Autodesk Inventor part; units mm, degrees
ref_plane "YZ Plane" through (0, 0, 0) normal (1, 0, 0) x (0, 1, 0)
ref_plane "XZ Plane" through (0, 0, 0) normal (0, 1, 0) x (-1, 0, 0)
ref_plane "XY Plane" through (0, 0, 0) normal (0, 0, 1) x (1, 0, 0)
sketch "Sketch1" plane through (0, 0, 0) normal (0, 0, 1) x (1, 0, 0)
  line L0 (0, 0) -> (25.4, 0)
  line L1 (25.4, 0) -> (25.4, 50.8)
  line L2 (25.4, 50.8) -> (0, 50.8)
  line L3 (0, 50.8) -> (0, 0)
  line L4 (1.5875, 1.5875) -> (23.8125, 1.5875)
  line L5 (23.8125, 1.5875) -> (23.8125, 49.2125)
  line L6 (23.8125, 49.2125) -> (1.5875, 49.2125)
  line L7 (1.5875, 49.2125) -> (1.5875, 1.5875)
  dimension "d0" = 25.4
  dimension "d1" = 50.8
  dimension "d2" = 1.5875
extrude "Extrusion1" add sketch "Sketch1" along normal blind 77.4446
sketch "Sketch2" plane through (25.4, 0, 0) normal (1, 0, 0) x (0, 0, -1)
  line L0 (0, 50.8) -> (-77.4446, 50.8)
  line L1 (-77.4446, 50.8) -> (-68.2676, 0)
  line L2 (-68.2676, 0) -> (-77.4446, 0)
  line L3 (0, 1.5875) -> (-77.4446, 1.5875)
  line L4 (-77.4446, 50.8) -> (-77.4446, 0)
  line L5 (-77.4446, 0) -> (-77.4446, 50.8)
  point P0 (0, 0)
  dimension "d5" = 10.24
sketch "Sketch3" plane through (25.4, 0, 0) normal (1, 0, 0) x (0, 0, -1)
  line L0 (0, 0) -> (0, 50.8)
  line L1 (0, 50.8) -> (-77.4446, 50.8)
  line L2 (-77.4446, 0) -> (-77.4446, 50.8)
  point P0 (-26.797, 25.4)
  dimension "d10" = 25.4
  dimension "d21" = 50.6476
hole "Hole1" at (25.4, 25.4, 26.797) direction (-1, 0, 0) diameter 28.575 depth 25.4 tip angle 118
extrude "Extrusion3" cut sketch "Sketch2" against normal blind 25.4
properties part number "ARM_029_BottomIntakeSide" material "Aluminum 6061"
Read the model definition and answer for the solid it produces. Units are mm, in the model's axes. A direction names the side the tool comes from. Coordinates: 2 decimals unless noted, no trailing zeros. Write each loop counter-clockwise with the first axis right and the second up, starting at its lowest first coordinate (ties: lowest second). Pieces come first, ordered by that corner, then holes. Notation, with made-up numbers: (18.5, -29) - (23.5, -29) arc R21 cw to (23.5, -11) - close; hole circle Ø6 at (27.25, -5). An arc over 180 degrees is marked (long way). Answer as a JSON object with one key per item and string values. Group by question number.
1. A cutting plane is placed at C-C (y = 25.4). Determine the outline of the cut face in (x, z), plus the area to 3 significant figures.
2. Which of the six approach directions +Z, -Z, +X, -X, +Y, -Y give full straight-line access (tool end or side, diameter ignored) to faces 5 (the cylindrical face through (0.783, 11.234, 28.657)), 6 (the flat face through (13, 1.588, 34))?
3. This flat-tipped pin is pushed along its axis until it touches: P1, Ø6, axis at y = 36.5, z = 24, coming from the -X side. Where does it stop, or does it pass through?
4. A cutting plane is placed at A-A (x = 4). Determine the outline of the cut face in (y, z).
5. Consider L1, parallel to Y at x = 13, z = 23; L2, parallel to X at y = 4, z = 32.5; L3, parallel to Z at x = 0.7, y = 25.4. Determine where each line is inside the solid, lowest interval first. Write a range as [from, to].
6. A cutting plane is placed at B-B (z = 56.5). Determine the outline of the cut face in (x, y), plus the area to 3 significant figures.
7. A cutting plane is placed at D-D (z = 26.5). Determine the outline of the cut face in (x, y), plus the area to 3 significant figures.
8. The mould has two halves that part along Y. Classify faces 1 (the flat face through (25.4, 25, 47)), 2 (the flat face through (13, 49.212, 38)), 3 (the flat face through (23.812, 25, 47)), 4 (the flat face through (0.53, 25.519, 72.878)): +Y half, -Y half, draft (parallel to the pull), parting line (faces both ways), or undercut.
Worked out:
{
 "1": {"outline": "(0, 0) - (1.59, 0) - (1.59, 12.51) - (0, 12.51) - close; (0, 41.08) - (1.59, 41.08) - (1.59, 72.86) - (0, 72.86) - close; (23.81, 0) - (25.4, 0) - (25.4, 12.51) - (23.81, 12.51) - close; (23.81, 41.08) - (25.4, 41.08) - (25.4, 72.86) - (23.81, 72.86) - close", "area": "141 mm²"},
 "2": {"face 5": "+X, -X", "face 6": "+Z, -Z"},
 "3": {"P1": "stops at x = 0"},
 "4": {"outline": "(0, 0) - (1.59, 0) - (1.59, 68.55) - (0, 68.27) - close; (49.21, 0) - (50.8, 0) - (50.8, 77.44) - (49.21, 77.16) - close"},
 "5": {"L1": "y = [0, 1.59], [49.21, 50.8]", "L2": "x = [0, 1.59], [23.81, 25.4]", "L3": "z = [0, 12.51], [41.08, 72.86]"},
 "6": {"outline": "(0, 0) - (25.4, 0) - (25.4, 50.8) - (0, 50.8) - close; hole (1.59, 1.59) - (23.81, 1.59) - (23.81, 49.21) - (1.59, 49.21) - close", "area": "232 mm²"},
 "7": {"outline": "(0, 0) - (25.4, 0) - (25.4, 11.12) - (23.81, 11.12) - (23.81, 1.59) - (1.59, 1.59) - (1.59, 11.12) - (0, 11.12) - close; (0, 39.68) - (1.59, 39.68) - (1.59, 49.21) - (23.81, 49.21) - (23.81, 39.68) - (25.4, 39.68) - (25.4, 50.8) - (0, 50.8) - close", "area": "141 mm²"},
 "8": {"face 1": "draft", "face 2": "undercut", "face 3": "undercut", "face 4": "-Y half"}
}
